The model under review builds one solid part; all positions refer to its coordinate system, in mm. Face numbers are marked on the shaded views. A direction names the side the tool comes from. Round coordinates to 2 decimals unless told otherwise and drop trailing zeros. Write each loop counter-clockwise with the first axis right and the second up, starting at its lowest first coordinate (ties: lowest second). Pieces come first, ordered by that corner, then holes. Notation, with made-up numbers: M 81.25,41.5 L 121.25,41.5 A8 ccw 121.25,46.5 Z; hole C 52,-34.5 d2. An arc over 180 degrees is marked long. One line per item, written item: value. Start each with the question number.
1) Take a section at C-C, the plane y = -78. Write out the cut boundary in (x, z), and give its area (3 significant figures).
2) For P1, Ø1, axis at y = 6.5, z = -1.5, coming from the +X side; P2, Ø6, axis at y = 4, z = 0.5, coming from the +X side; P3, Ø6, axis at x = -12.5, z = -4, coming from the +Y side; P4, Ø2, axis at x = -11.5, y = -49, coming from the +Z side, all flat-tipped, find the tip position at first contact; note any pin that passes through.
3) Mouldability with a two-part tool opening along X and no side actions: class the marked faces 1, 2 and 3 as +X half, -X half, draft (parallel to the pull), parting line (faces both ways), or undercut.
4) Tool access review of the marked faces 4 and 5: name each direction out of +Z, -Z, +X, -X, +Y, -Y from which nothing blocks a thin tool from reaching the whole face with its end or side.
5) Wall thickness on probe 1 along Y at (x, z) = (-12, -15); probe 2 along X at (y, z) = (-43.5, 3); probe 3 along X at (y, z) = (0, -1): over which ranges is each line inside the solid? List them lowest first.
6) Take a section at B-B, the plane z = 0. Write out the cut boundary in (x, y), and give its area (3 significant figures).
7) Take a section at A-A, the plane x = 0. Write out the cut boundary in (y, z), and give its area (3 significant figures).
8) Take a section at D-D, the plane y = -37. Write out the cut boundary in (x, z), and give its area (3 significant figures).
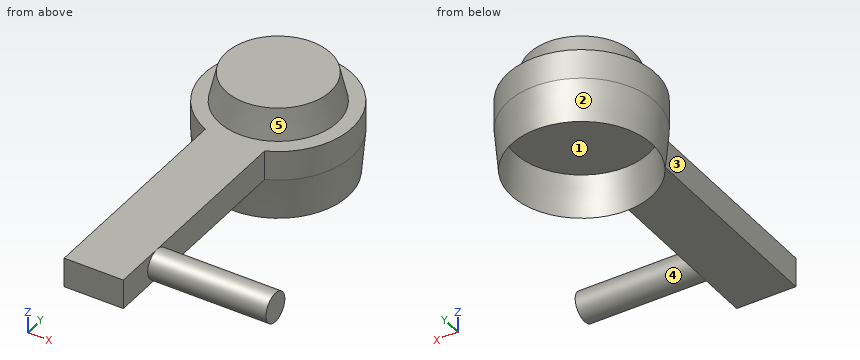
from build123d import *

# Parameters (mm, degrees)
BOSS_EXTRUDE1_DEPTH = 5
SKETCH2_R           = 20
BOSS_EXTRUDE2_DEPTH = 10
BOSS_EXTRUDE2_TAPER = 13
SKETCH3_R           = 25
SKETCH3_R_2         = 22.5
BOSS_EXTRUDE3_DEPTH = 15
BOSS_EXTRUDE3_TAPER = 5
SKETCH4_R           = 5
BOSS_EXTRUDE4_DEPTH = 40


with BuildPart() as part:
    # Sketch1 → Boss-Extrude1 (new, symmetric)
    with BuildSketch(Plane.XY):
        with BuildLine():
            Line((-10, -22.912878475), (-10, -97.912878475))
            Line((-10, -97.912878475), (10, -97.912878475))
            Line((10, -97.912878475), (10, -22.912878475))
            ThreePointArc((10, -22.912878475), (0, 25), (-10, -22.912878475))
        make_face()
    extrude(amount=BOSS_EXTRUDE1_DEPTH, both=True)

    # Sketch2 → Boss-Extrude2 (add)
    with BuildSketch(Plane.XY.offset(5)):
        Circle(SKETCH2_R)
    extrude(amount=BOSS_EXTRUDE2_DEPTH, taper=BOSS_EXTRUDE2_TAPER)

    # Sketch3 → Boss-Extrude3 (add)
    with BuildSketch(Plane(origin=(0, 0, -5), x_dir=(-1, 0, 0), z_dir=(0, 0, -1))):
        Circle(SKETCH3_R)
        Circle(SKETCH3_R_2, mode=Mode.SUBTRACT)
    extrude(amount=BOSS_EXTRUDE3_DEPTH, taper=BOSS_EXTRUDE3_TAPER)

    # Sketch4 → Boss-Extrude4 (add)
    with BuildSketch(Plane(origin=(10, 0, 0), x_dir=(0, 0, -1), z_dir=(1, 0, 0))):
        with Locations((0, -80)):
            Circle(SKETCH4_R)
    extrude(amount=BOSS_EXTRUDE4_DEPTH)


solid = part.part
Checked values:
1. outline: M -10,-5 L 10,-5 L 10,-4.58 L 50,-4.58 L 50,4.58 L 10,4.58 L 10,5 L -10,5 Z
1. area: 567 mm2
2. P1: stops at x = 24.27
2. P2: stops at x = 24.98
2. P3: stops at y = 23.12
2. P4: passes through
3. face 1: undercut
3. face 2: parting line
3. face 3: -X half
4. face 4: +X
4. face 5: +Z
5. probe 1: y = -20.93 to -20.06, 20.06 to 20.93
5. probe 2: x = -10 to 10
5. probe 3: x = -25 to 25
6. outline: M -10,-97.91 L 10,-97.91 L 10,-85 L 50,-85 L 50,-75 L 10,-75 L 10,-22.91 A25 ccw long -10,-22.91 Z
6. area: 3,840 mm2
7. outline: M -97.91,-5 L -25,-5 L -23.75,-19.29 L -22.5,-5 L 22.5,-5 L 23.75,-19.29 L 25,-5 L 25,5 L 20,5 L 17.69,15 L -17.69,15 L -20,5 L -97.91,5 Z
7. area: 1,640 mm2
8. outline: M -10,-5 L 10,-5 L 10,5 L -10,5 Z
8. area: 200 mm2
